Job drawing, mm, ordinate dimensions from the low corner. One solid piece. Round coordinates to 2 decimals unless told otherwise and drop trailing zeros. Loops run counter-clockwise (first coordinate to the right, second up) from the corner with the lowest first, then second, coordinate; pieces in that order, holes last.
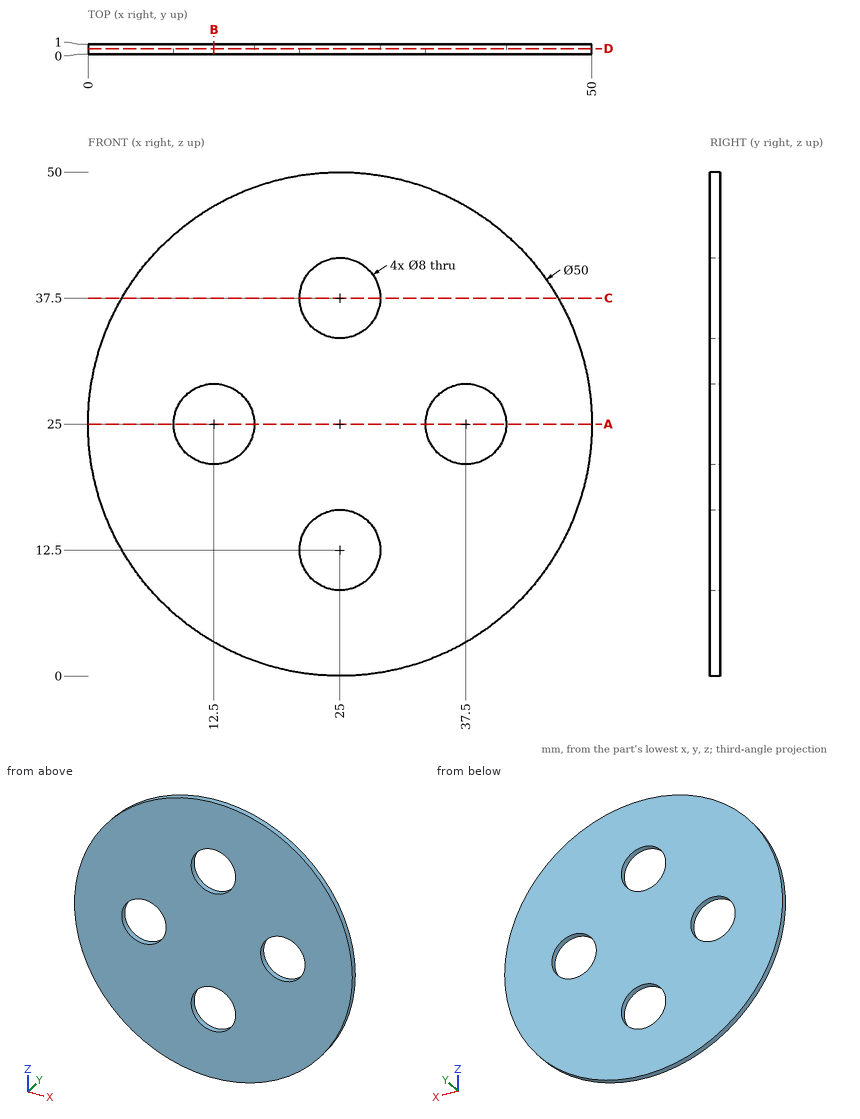
1) Slice it at C-C, the plane z = 37.5. Give the cut face in (x, y).
Values:
outline: (3.35, 0) - (21, 0) - (21, 1) - (3.35, 1) - close; (29, 0) - (46.65, 0) - (46.65, 1) - (29, 1) - close
2) Wall check: line 1 along Z through (x, y) = (25, 0.2); line 2 along X through (y, z) = (0.6, 26). Give the ranges that are in metal, low to high.
Values:
line 1: z = 0 to 8.5, 16.5 to 33.5, 41.5 to 50
line 2: x = 0.02 to 8.63, 16.37 to 33.63, 41.37 to 49.98
3) Slice it at D-D, the plane y = 0.55. Give the cut face in (x, z).
Values:
outline: circle Ø50 at (25, 25); hole circle Ø8 at (12.5, 25); hole circle Ø8 at (25, 12.5); hole circle Ø8 at (25, 37.5); hole circle Ø8 at (37.5, 25)
4) Slice it at A-A, the plane z = 25. Give the cut face in (x, y).
Values:
outline: (0, 0) - (8.5, 0) - (8.5, 1) - (0, 1) - close; (16.5, 0) - (33.5, 0) - (33.5, 1) - (16.5, 1) - close; (41.5, 0) - (50, 0) - (50, 1) - (41.5, 1) - close
5) Slice it at B-B, the plane x = 12.5. Give the cut face in (y, z), then the cut area to 3 significant figures.
Values:
outline: (0, 3.35) - (1, 3.35) - (1, 21) - (0, 21) - close; (0, 29) - (1, 29) - (1, 46.65) - (0, 46.65) - close
area: 35.3 mm2
